Geometry check sheet. Reference: the model listing, model coordinates, mm. Face numbers are marked on the shaded views. A direction names the side the tool comes from. Round coordinates to 2 decimals unless told otherwise and drop trailing zeros. Write each loop counter-clockwise with the first axis right and the second up, starting at its lowest first coordinate (ties: lowest second). Pieces come first, ordered by that corner, then holes. Notation, with made-up numbers: M 69.5,18.5 L 97.5,18.5 A25 cw 97.5,34.5 Z; hole C 3.5,26 d3. An arc over 180 degrees is marked long. Use a Markdown table: item, result.
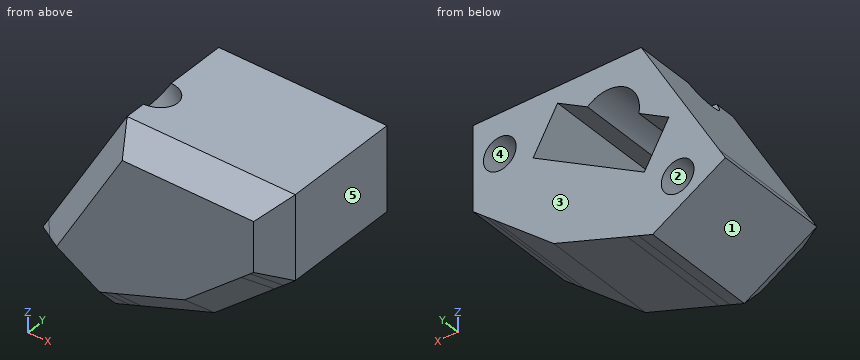
Autodesk Inventor part; units mm, degrees
ref_plane "YZ Plane" through (0, 0, 0) normal (1, 0, 0) x (0, 1, 0)
ref_plane "XZ Plane" through (0, 0, 0) normal (0, 1, 0) x (-1, 0, 0)
ref_plane "XY Plane" through (0, 0, 0) normal (0, 0, 1) x (1, 0, 0)
sketch "Sketch1" plane through (0, 0, 0) normal (0, 1, 0) x (-1, 0, 0)
  line L0 (50.7332, 97.4522) -> (55.4964, 94.7022)
  line L1 (55.4964, 94.7022) -> (57.5964, 98.3395)
  line L2 (48.0701, 103.8395) -> (45.9701, 100.2022)
  line L3 (45.9701, 100.2022) -> (50.7332, 97.4522)
  arc A0 (55.0378, 99.8167) -> (50.6287, 102.3623) centre (52.3832, 100.3101) ccw
  line L4 (48.0701, 103.8395) -> (50.6287, 102.3623)
  line L5 (55.0378, 99.8167) -> (57.5964, 98.3395)
  line L6 (47.7332, 92.256) -> (54.0309, 89.9639)
  line L7 (47.7332, 92.256) -> (54.435, 92.256) construction
  line L8 (56.5464, 96.5209) -> (59.5464, 96.5209) construction
  line L9 (58.0464, 93.9228) -> (60.2464, 93.9228) construction
  line L10 (54.0309, 89.9639) -> (54.9868, 89.616)
  line L11 (55.2332, 105.2464) -> (61.9398, 93.6303)
  circle A1 centre (58.3542, 93.0522) radius 1.4
  line L12 (61.9398, 93.6303) -> (62.4398, 92.7643)
  line L13 (62.4398, 92.7643) -> (56.2134, 89.1695)
  line L14 (54.9868, 89.616) -> (56.2134, 89.1695)
  line L15 (47.7332, 92.256) -> (42.5993, 96.5639)
  line L16 (47.7332, 92.256) -> (44.3823, 98.06) construction
  line L17 (47.0201, 102.0209) -> (45.5201, 104.6189) construction
  line L18 (44.0201, 102.0209) -> (42.9201, 103.9261) construction
  line L19 (42.5993, 96.5639) -> (41.8201, 97.2178)
  line L20 (55.2332, 105.2464) -> (41.8201, 105.2464)
  circle A2 centre (43.1122, 101.8522) radius 1.4
  line L21 (41.8201, 105.2464) -> (40.8201, 105.2464)
  line L22 (40.8201, 105.2464) -> (40.8201, 98.0569)
  line L23 (41.8201, 97.2178) -> (40.8201, 98.0569)
  dimension "d8" = 20
  dimension "d26" = 2.8
  dimension "d27" = 1
  dimension "d31" = 2.8
extrude "Extrusion1" add sketch "Sketch1" along normal blind 12
sketch "Sketch3" plane through (0, 0, 0) normal (0, -1, 0) x (1, 0, 0)
  line L0 (-48.0701, 103.8395) -> (-45.9701, 100.2022)
  line L1 (-45.9701, 100.2022) -> (-55.4964, 94.7022)
  line L2 (-55.4964, 94.7022) -> (-57.5964, 98.3395)
  line L3 (-57.5964, 98.3395) -> (-55.0378, 99.8167)
  arc A0 (-50.6287, 102.3623) -> (-55.0378, 99.8167) centre (-52.3832, 100.3101) ccw
  line L4 (-50.6287, 102.3623) -> (-48.0701, 103.8395)
  line L5 (-55.2332, 105.2464) -> (-62.4398, 92.7643)
  line L6 (-56.2134, 89.1695) -> (-47.7332, 92.256)
  line L7 (-62.4398, 92.7643) -> (-56.2134, 89.1695)
  line L8 (-47.7332, 92.256) -> (-40.8201, 98.0569)
  line L9 (-40.8201, 98.0569) -> (-40.8201, 105.2464)
  line L10 (-40.8201, 105.2464) -> (-55.2332, 105.2464)
  circle A1 centre (-58.3542, 93.0522) radius 1.4
  circle A2 centre (-43.1122, 101.8522) radius 1.4
  point P0 (0, 0)
extrude "Extrusion2" add sketch "Sketch3" against normal blind 2 contours L0 L1 L2 L3 A0 L4 | A1 | A2
sketch "Sketch4" plane through (-45.9701, 2, 100.2022) normal (-0.5, 0, 0.8660254) x (0.8660254, 0, 0.5)
  line L0 (0, 0) -> (-5.5, 0)
  line L1 (-11, 0) -> (0, 0)
  line L2 (-5.5, 0) -> (-5.5, 3.3)
  circle A0 centre (-5.5, 3.3) radius 1.5
  point P0 (-10.2898, -2)
  dimension "d21" = 3.3
  dimension "d22" = 3
extrude "Extrusion3" cut sketch "Sketch4" along normal through all
chamfer "Chamfer2" distance 2 angle 45 6 edges at (-58.8365, 0, 99.0054) (-48.0267, 0, 105.2464) (-40.8201, 0, 101.6516) (-44.2767, 0, 95.1565) (-51.9733, 0, 90.7128) (-59.3266, 0, 90.9669)
properties part number "TSOP Holder Corner" material "ABS Plastic"
Item 1: Cross-section at D-D, the plane z = 90.5. Record the cut outline in (x, y).
Outcome:
| item | result |
|---|---|
| outline | M -58.52,2 L -56.1,0.79 L -55.31,1.06 L -54.23,1.43 L -52.56,2 L -52.56,12 L -58.52,12 Z |
Item 2: Cross-section at C-C, the plane y = 8.25. Record the cut outline in (x, z), and give its area (3 significant figures).
Outcome:
| item | result |
|---|---|
| outline | M -62.44,92.76 L -56.21,89.17 L -54.99,89.62 L -54.03,89.96 L -47.73,92.26 L -42.6,96.56 L -41.82,97.22 L -40.82,98.06 L -40.82,105.25 L -55.23,105.25 L -61.94,93.63 Z; hole C -58.35,93.05 d2.8; hole M -57.6,98.34 L -55.5,94.7 L -50.73,97.45 L -45.97,100.2 L -48.07,103.84 L -50.63,102.36 A2.7 ccw -55.04,99.82 Z; hole C -43.11,101.85 d2.8 |
| area | 172 mm2 |
Item 3: Access from +Z, -Z, +X, -X, +Y, -Y to the whole of each face (thin tool, end or side, straight path). Record for the marked faces 1 and 2.
Outcome:
| item | result |
|---|---|
| face 1 | -Z, -X, +Y, -Y |
| face 2 | +Y |
Item 4: Cross-section at B-B, the plane x = -57.25. Record the cut outline in (y, z), and give its area (3 significant figures).
Outcome:
| item | result |
|---|---|
| outline | M 0,92.08 L 2,89.77 L 12,89.77 L 12,92.19 L 2,92.19 L 2,93.91 L 12,93.91 L 12,97.74 L 2,97.74 L 2,98.54 L 12,98.54 L 12,101.75 L 2,101.75 L 0,97.75 Z |
| area | 112 mm2 |
Item 5: Material ranges on line 1 along X through (y, z) = (8, 101.5); line 2 along Z through (x, y) = (-42.5, 10); line 3 along Z through (x, y) = (-52.25, 4.75), recorded low to high. Write a range as from..to.
Outcome:
| item | result |
|---|---|
| line 1 | x = -57.4..-54.81, -46.72..-44.47, -41.76..-40.82 |
| line 2 | z = 96.65..100.59, 103.11..105.25 |
| line 3 | z = 90.61..96.58, 103.01..105.25 |
Item 6: Go/stop test with flat-tipped pins: pin 1 (5 mm diameter, centred on y = 8.5, z = 97, fed in from -X); pin 2 (2.5 mm diameter, centred on x = -52, z = 99.5, fed in from +Y); pin 3 (1 mm diameter, centred on y = 5, z = 100, fed in from -X). Record where each tip stops, or that it passes through.
Outcome:
| item | result |
|---|---|
| pin 1 | stops at x = -61.44 |
| pin 2 | stops at y = 2 |
| pin 3 | stops at x = -58.55 |
Item 7: Cross-section at A-A, the plane y = 6. Record the cut outline in (x, z).
Outcome:
| item | result |
|---|---|
| outline | M -62.44,92.76 L -56.21,89.17 L -54.99,89.62 L -54.03,89.96 L -47.73,92.26 L -42.6,96.56 L -41.82,97.22 L -40.82,98.06 L -40.82,105.25 L -53.7,105.25 L -52.41,103.01 A2.7 cw -50.63,102.36 L -48.07,103.84 L -45.97,100.2 L -50.73,97.45 L -55.5,94.7 L -57.6,98.34 L -55.04,99.82 A2.7 cw -54.71,101.68 L -56,103.92 L -61.94,93.63 Z; hole C -58.35,93.05 d2.8; hole C -43.11,101.85 d2.8 |
Item 8: Mould release check, pull along X, two halves, no side actions. Record for the marked faces 3, 4 and 5: +X half, -X half, draft (parallel to the pull), parting line (faces both ways), or undercut.
Outcome:
| item | result |
|---|---|
| face 3 | draft |
| face 4 | undercut |
| face 5 | +X half |
